```python
from build123d import *

# Parameters (mm, degrees)
BOSS_EXTRUDE1_DEPTH = 58.9788
FILLET3_R           = 5.0292
SKETCH2_R           = 3.9878
SKETCH2_R_2         = 3.937
CUT_EXTRUDE1_DEPTH  = 58.9788
SKETCH3_R           = 4.6482
CUT_EXTRUDE6_DEPTH  = 3.0988
CUT_EXTRUDE6_TAPER  = 35
SKETCH5_R           = 4.6482
CUT_EXTRUDE7_DEPTH  = 3.0988
CUT_EXTRUDE7_TAPER  = 35
SKETCH6_R           = 3.9878
CUT_EXTRUDE8_DEPTH  = 50.8
SKETCH7_R           = 3.8862
CUT_EXTRUDE9_DEPTH  = 50.8


with BuildPart() as part:
    # Sketch1 → Boss-Extrude1 (new body)
    with BuildSketch(Plane.XY):
        with BuildLine():
            Line((0, 0), (3.3274, 0))
            ThreePointArc((3.3274, 0), (3.943440488, -0.07583805), (4.522694118, -0.298823529))
            Line((4.522694118, -0.298823529), (6.965576471, -1.601694118))
            ThreePointArc((6.965576471, -1.601694118), (7.544830101, -1.824679597), (8.160870588, -1.900517647))
            Line((8.160870588, -1.900517647), (21.498585253, -1.900517647))
            ThreePointArc((21.498585253, -1.900517647), (22.681569141, -1.96962328), (23.848460342, -2.176000104))
            Line((23.848460342, -2.176000104), (36.989870588, -5.300145762))
            Line((36.989870588, -5.300145762), (36.989870588, -2.27162931))
            Line((36.989870588, -2.27162931), (24.193875089, 0.770399896))
            ThreePointArc((24.193875089, 0.770399896), (23.026983888, 0.97677672), (21.844, 1.045882353))
            Line((21.844, 1.045882353), (8.897470588, 1.045882353))
            ThreePointArc((8.897470588, 1.045882353), (8.281430101, 1.121720403), (7.702176471, 1.344705882))
            Line((7.702176471, 1.344705882), (5.259294118, 2.647576471))
            ThreePointArc((5.259294118, 2.647576471), (4.680040488, 2.87056195), (4.064, 2.9464))
            Line((4.064, 2.9464), (-4.064, 2.9464))
            ThreePointArc((-4.064, 2.9464), (-4.680040488, 2.87056195), (-5.259294118, 2.647576471))
            Line((-5.259294118, 2.647576471), (-7.702176471, 1.344705882))
            ThreePointArc((-7.702176471, 1.344705882), (-8.281430101, 1.121720403), (-8.897470588, 1.045882353))
            Line((-8.897470588, 1.045882353), (-21.844, 1.045882353))
            ThreePointArc((-21.844, 1.045882353), (-23.026983888, 0.97677672), (-24.193875089, 0.770399896))
            Line((-24.193875089, 0.770399896), (-36.989870588, -2.27162931))
            Line((-36.989870588, -2.27162931), (-36.989870588, -5.300145762))
            Line((-36.989870588, -5.300145762), (-23.848460342, -2.176000104))
            ThreePointArc((-23.848460342, -2.176000104), (-22.681569141, -1.96962328), (-21.498585253, -1.900517647))
            Line((-21.498585253, -1.900517647), (-8.160870588, -1.900517647))
            ThreePointArc((-8.160870588, -1.900517647), (-7.544830101, -1.824679597), (-6.965576471, -1.601694118))
            Line((-6.965576471, -1.601694118), (-4.522694118, -0.298823529))
            ThreePointArc((-4.522694118, -0.298823529), (-3.943440488, -0.07583805), (-3.3274, 0))
            Line((-3.3274, 0), (0, 0))
        make_face()
    extrude(amount=BOSS_EXTRUDE1_DEPTH)

    # Fillet3
    fillet3_edges = [part.edges().sort_by_distance(p)[0] for p in [
        (-36.989870588, -3.785887536, 0),
        (36.989870588, -3.785887536, 0),
        (36.989870588, -3.785887536, 58.9788),
        (-36.989870588, -3.785887536, 58.9788),
    ]]
    fillet(fillet3_edges, radius=FILLET3_R)

    # Sketch2 → Cut-Extrude1 (cut)
    with BuildSketch(Plane(origin=(-1.467570487, 6.173190353, 0), x_dir=(0.972885585, 0.231286918, 0), z_dir=(-0.231286918, 0.972885585, 0))):
        with Locations((-27.927110028, -10.1854)):
            Circle(SKETCH2_R)
        with Locations((-27.927110028, -29.4894)):
            Circle(SKETCH2_R_2)
        with Locations((-27.927110028, -48.8188)):
            Circle(SKETCH2_R)
    extrude(amount=-CUT_EXTRUDE1_DEPTH, mode=Mode.SUBTRACT)

    # Sketch3 → Cut-Extrude6 (cut)
    with BuildSketch(Plane(origin=(0, 1.045882353, 0), x_dir=(1, 0, 0), z_dir=(0, 1, 0))):
        with Locations((-15.24, -10.668)):
            Circle(SKETCH3_R)
        with Locations((-15.24, -23.368)):
            Circle(SKETCH3_R)
        with Locations((-15.24, -36.068)):
            Circle(SKETCH3_R)
        with Locations((-15.24, -48.768)):
            Circle(SKETCH3_R)
    extrude(amount=-CUT_EXTRUDE6_DEPTH, taper=CUT_EXTRUDE6_TAPER, mode=Mode.SUBTRACT)

    # Sketch5 → Cut-Extrude7 (cut)
    with BuildSketch(Plane(origin=(0, 1.045882353, 0), x_dir=(1, 0, 0), z_dir=(0, 1, 0))):
        with Locations((15.24, -10.668)):
            Circle(SKETCH5_R)
        with Locations((15.24, -23.368)):
            Circle(SKETCH5_R)
        with Locations((15.24, -36.068)):
            Circle(SKETCH5_R)
        with Locations((15.24, -48.768)):
            Circle(SKETCH5_R)
    extrude(amount=-CUT_EXTRUDE7_DEPTH, taper=CUT_EXTRUDE7_TAPER, mode=Mode.SUBTRACT)

    # Sketch6 → Cut-Extrude8 (cut)
    with BuildSketch(Plane(origin=(1.467570487, 6.173190353, 0), x_dir=(0.972885585, -0.231286918, 0), z_dir=(0.231286918, 0.972885585, 0))):
        with Locations((27.876310028, -10.16)):
            Circle(SKETCH6_R)
        with Locations((27.876310028, -29.464)):
            Circle(SKETCH6_R)
        with Locations((27.876310028, -48.768)):
            Circle(SKETCH6_R)
    extrude(amount=-CUT_EXTRUDE8_DEPTH, mode=Mode.SUBTRACT)

    # Sketch7 → Cut-Extrude9 (cut)
    with BuildSketch(Plane(origin=(0, 2.9464, 0), x_dir=(1, 0, 0), z_dir=(0, 1, 0))):
        with Locations((0, -10.16)):
            Circle(SKETCH7_R)
        with Locations((0, -29.5148)):
            Circle(SKETCH7_R)
        with Locations((0, -48.8696)):
            Circle(SKETCH7_R)
    extrude(amount=-CUT_EXTRUDE9_DEPTH, mode=Mode.SUBTRACT)


solid = part.part
```
Input: part model. Units: mm. Frame: model coordinates. A direction names the side the tool comes from. Coordinates: 2 decimals unless noted, no trailing zeros. Loops run counter-clockwise (first coordinate to the right, second up) from the corner with the lowest first, then second, coordinate; pieces in that order, holes last. Notation, with made-up numbers: M -36.75,45 L -30.75,45 A19 ccw -30.75,50 Z; hole C 29.25,-32.75 d4. An arc over 180 degrees is marked long. One line per item, written item: value.
(1) Section D-D (x = -28). Give the number of separate pieces and of enclosed holes in the cut face, and give its area (3 significant figures).
Filled in:
separate pieces: 4
enclosed holes: 0
area: 107 mm^2
(2) Section C-C (z = 55). Output: boundary loops of the cut face in (x, y), and give its area (3 significant figures).
Filled in:
outline: M -36.88,-5.27 L -23.85,-2.18 A10.16 cw -21.5,-1.9 L -8.16,-1.9 A2.54 ccw -6.97,-1.6 L -4.52,-0.3 A2.54 cw -3.33,0 L 3.33,0 A2.54 cw 4.52,-0.3 L 6.97,-1.6 A2.54 ccw 8.16,-1.9 L 21.5,-1.9 A10.16 cw 23.85,-2.18 L 36.88,-5.27 L 36.88,-2.25 L 24.19,0.77 A10.16 ccw 21.84,1.05 L 8.9,1.05 A2.54 cw 7.7,1.34 L 5.26,2.65 A2.54 ccw 4.06,2.95 L -4.06,2.95 A2.54 ccw -5.26,2.65 L -7.7,1.34 A2.54 cw -8.9,1.05 L -21.84,1.05 A10.16 ccw -24.19,0.77 L -36.88,-2.25 Z
area: 222 mm^2
(3) Section B-B (x = -15.24). Output: boundary loops of the cut face in (y, z), and give its area (3 significant figures).
Filled in:
outline: M -1.9,0 L 1.05,0 L 1.05,6.02 L -1.9,8.08 Z; M -1.9,13.25 L 1.05,15.32 L 1.05,18.72 L -1.9,20.78 Z; M -1.9,25.95 L 1.05,28.02 L 1.05,31.42 L -1.9,33.48 Z; M -1.9,38.65 L 1.05,40.72 L 1.05,44.12 L -1.9,46.18 Z; M -1.9,51.35 L 1.05,53.42 L 1.05,58.98 L -1.9,58.98 Z
area: 88.5 mm^2
(4) Reachability of faces 4 (the cylindrical face through (-35.556, -3.218, 57.466)), 5 (the flat face through (-15, -1.901, 29)) from +Z, -Z, +X, -X, +Y, -Y: full face, straight path, thin tool, end or side. Return the list, or none.
Filled in:
face 4: +Z, -X, +Y, -Y
face 5: +Z, -Z, -Y
(5) Pull-direction query (X, two-part tool) for faces 1 (the flat face through (15, 1.046, 29)), 2 (the flat face through (-31.971, -4.107, 29.077)), 3 (the flat face through (-33.346, -1.405, 29.077)); classes: +X half, -X half, draft (parallel to the pull), parting line (faces both ways), or undercut.
Filled in:
face 1: draft
face 2: undercut
face 3: -X half
(6) Line query: line 1 along Z through (x, y) = (0, 1.3); line 2 along Z through (x, y) = (-15, -1.5); line 3 along X through (y, z) = (0.25, 48.5). Output: solid intervals per line, ascending. Write a range as from..to.
Filled in:
line 1: 0..6.27, 14.05..25.63, 33.4..44.98, 52.76..58.98
line 2: 0..7.81, 13.52..20.51, 26.22..33.21, 38.92..45.91, 51.62..58.98
line 3: -24.68..-19.32, -11.16..-3.87, 3.87..11.16, 19.32..24.62
(7) Section A-A (x = 0). Output: boundary loops of the cut face in (y, z), and give its area (3 significant figures).
Filled in:
outline: M 0,0 L 2.95,0 L 2.95,6.27 L 0,6.27 Z; M 0,14.05 L 2.95,14.05 L 2.95,25.63 L 0,25.63 Z; M 0,33.4 L 2.95,33.4 L 2.95,44.98 L 0,44.98 Z; M 0,52.76 L 2.95,52.76 L 2.95,58.98 L 0,58.98 Z
area: 105 mm^2
(8) Pin query (flat end, axial travel): pin 1 (6 mm diameter, centred on x = -29, z = 31, fed in from +Y); pin 2 (4 mm diameter, centred on x = 14, z = 19, fed in from +Y); pin 3 (10 mm diameter, centred on x = 0, z = 10.16, fed in from -Y); pin 4 (6 mm diameter, centred on x = 0, z = 48.87, fed in from +Y). Return the tip coordinate at first contact, or that it passes through.
Filled in:
pin 1: y = 0.19
pin 2: y = 1.05
pin 3: y = -0.55
pin 4: through
